```python
from build123d import *

# Parameters (mm, degrees)
BOSS_EXTRUDE1_DEPTH = 12
SKETCH2_R           = 3.1
BOSS_EXTRUDE2_DEPTH = 15
CUT_EXTRUDE1_START  = -50
CUT_EXTRUDE1_DEPTH  = 50
CUT_EXTRUDE2_START  = -15
CUT_EXTRUDE2_DEPTH  = 15
SKETCH5_W           = 7
SKETCH5_H           = 112.5
CUT_EXTRUDE3_DEPTH  = 12
SKETCH6_R           = 5.15
CUT_EXTRUDE4_DEPTH  = 2
FILLET1_R           = 4
BOSS_EXTRUDE3_DEPTH = 10
SKETCH9_R           = 2.1
CUT_EXTRUDE5_DEPTH  = 7
BOSS_EXTRUDE4_DEPTH = 7
SKETCH11_W          = 3.391399245
SKETCH11_H          = 0.49647288
BOSS_EXTRUDE7_DEPTH = 7
BOSS_EXTRUDE8_DEPTH = 10


with BuildPart() as part:
    # Sketch1 → Boss-Extrude1 (new body)
    with BuildSketch(Plane.XY):
        with BuildLine():
            Line((-5.64516129, 102.580645161), (-5.64516129, -27.419354839))
            ThreePointArc((-5.64516129, -27.419354839), (1.85483871, -34.919354839), (9.35483871, -27.419354839))
            Line((9.35483871, -27.419354839), (9.35483871, 102.580645161))
            ThreePointArc((9.35483871, 102.580645161), (1.85483871, 110.080645161), (-5.64516129, 102.580645161))
        make_face()
    extrude(amount=BOSS_EXTRUDE1_DEPTH)

    # Sketch2 → Boss-Extrude2 (add)
    with BuildSketch(Plane.XY.offset(12)):
        with Locations(Location((1.85483871, -27.419354839, 0), (0, 0, 180))):
            Circle(SKETCH2_R)
    extrude(amount=BOSS_EXTRUDE2_DEPTH)

    # Sketch3 → Cut-Extrude1 (cut)
    with BuildSketch(Plane.XY.offset(27).offset(CUT_EXTRUDE1_START)):
        with BuildLine():
            Line((0.166644408, -24.819354839), (3.543033011, -24.819354839))
            ThreePointArc((3.543033011, -24.819354839), (1.85483871, -30.519354839), (0.166644408, -24.819354839))
        make_face()
    extrude(amount=CUT_EXTRUDE1_DEPTH, mode=Mode.SUBTRACT)

    # Sketch4 → Cut-Extrude2 (cut)
    with BuildSketch(Plane.XY.offset(27).offset(CUT_EXTRUDE2_START)):
        with BuildLine():
            Line((0.166644408, -24.819354839), (3.543033011, -24.819354839))
            ThreePointArc((3.543033011, -24.819354839), (1.85483871, -24.319354839), (0.166644408, -24.819354839))
        make_face()
    extrude(amount=CUT_EXTRUDE2_DEPTH, mode=Mode.SUBTRACT)

    # Sketch5 → Cut-Extrude3 (cut)
    with BuildSketch(Plane.XY.offset(12)):
        with Locations((1.85483871, 36.330645161)):
            Rectangle(SKETCH5_W, SKETCH5_H)
    extrude(amount=-CUT_EXTRUDE3_DEPTH, mode=Mode.SUBTRACT)

    # Sketch6 → Cut-Extrude4 (cut)
    with BuildSketch(Plane.ZY.offset(5.64516129)):
        with Locations(Location((6, 78.768969581, 0), (0, 0, 270))):
            Circle(SKETCH6_R)
        with Locations(Location((6, 53.768969581, 0), (0, 0, 270))):
            Circle(SKETCH6_R)
        with Locations(Location((6, 28.768969581, 0), (0, 0, 270))):
            Circle(SKETCH6_R)
    extrude(amount=-CUT_EXTRUDE4_DEPTH, mode=Mode.SUBTRACT)

    # Fillet1
    # the kernel refuses this fillet: 4 mm, written as the material it adds along each edge
    with BuildSketch(Plane(origin=(-1.64516129, -19.919354839, 12), x_dir=(0, 1, 0), z_dir=(0, 0, -1)), Plane(origin=(5.35483871, -19.919354839, 12), x_dir=(-1, 0, 0), z_dir=(0, 0, -1)), Plane(origin=(5.35483871, 92.580645161, 12), x_dir=(0, -1, 0), z_dir=(0, 0, -1))) as fillet1_piece_1:
        with BuildLine():
            CenterArc((FILLET1_R, FILLET1_R), FILLET1_R, 180, 90)
            Line((0, FILLET1_R), (0, 0))
            Line((0, 0), (FILLET1_R, 0))
        make_face()
    extrude(amount=12)
    with BuildSketch(Plane(origin=(-1.64516129, 92.580645161, 12), x_dir=(0, -1, 0), z_dir=(0, 0, -1))) as fillet1_piece_2:
        with BuildLine():
            CenterArc((FILLET1_R, -FILLET1_R), FILLET1_R, 90, 90)
            Line((0, -FILLET1_R), (0, 0))
            Line((0, 0), (FILLET1_R, 0))
        make_face()
    extrude(amount=12)

    # Sketch7 → Boss-Extrude3 (add)
    with BuildSketch(Plane.XY.offset(12)):
        with BuildLine():
            ThreePointArc((-5.64516129, -27.419354839), (1.85483871, -34.919354839), (9.35483871, -27.419354839))
            ThreePointArc((9.35483871, -27.419354839), (1.85483871, -19.919354839), (-5.64516129, -27.419354839))
        make_face()
    extrude(amount=BOSS_EXTRUDE3_DEPTH)

    # Sketch9 → Cut-Extrude5 (cut)
    with BuildSketch(Plane.XY.offset(22)):
        with Locations((1.85483871, -27.419354839)):
            Circle(SKETCH9_R)
    extrude(amount=-CUT_EXTRUDE5_DEPTH, mode=Mode.SUBTRACT)

    # Sketch10 → Boss-Extrude4 (add)
    with BuildSketch(Plane.XY.offset(22)):
        with BuildLine():
            Line((0.694020033, -25.669354839), (3.015657386, -25.669354839))
            ThreePointArc((3.015657386, -25.669354839), (1.85483871, -25.319354839), (0.694020033, -25.669354839))
        make_face()
    extrude(amount=-BOSS_EXTRUDE4_DEPTH)

    # Sketch11 → Boss-Extrude7 (add)
    with BuildSketch(Plane.XY.offset(22)):
        with Locations((1.841860982, -25.665070635)):
            Rectangle(SKETCH11_W, SKETCH11_H)
    extrude(amount=-BOSS_EXTRUDE7_DEPTH)

    # Sketch12 → Boss-Extrude8 (add)
    with BuildSketch(Plane.XY.offset(22)):
        with BuildLine():
            Line((0.39134285, -25.913307075), (3.31833457, -25.913307075))
            ThreePointArc((3.31833457, -25.913307075), (1.85483871, -29.519354839), (0.39134285, -25.913307075))
        make_face()
        with BuildLine():
            Line((3.281340981, -26.003307075), (0.428336439, -26.003307075))
            ThreePointArc((0.428336439, -26.003307075), (1.85483871, -29.429354839), (3.281340981, -26.003307075))
        make_face(mode=Mode.SUBTRACT)
    extrude(amount=-BOSS_EXTRUDE8_DEPTH)


solid = part.part
```
Here's how the part is built. I have some questions about the finished solid (model axes, mm). A direction names the side the tool comes from. Round coordinates to 2 decimals unless told otherwise and drop trailing zeros. Write each loop counter-clockwise with the first axis right and the second up, starting at its lowest first coordinate (ties: lowest second). Pieces come first, ordered by that corner, then holes.
Q1. If we section it at B-B on z = 6: Write out the boundary of the cut face in (x, y), plus the area to 3 significant figures.
Q2. Which directions (+Z, -Z, +X, -X, +Y, -Y) give clear straight access to the entire face, cutting with the end or side of a thin tool? Please do faces 5 (the flat face through (5.355, 36, 6)), 6 (the flat face through (2, -28, 12)), 7 (the cylindrical face through (-4.659, 58.914, 6.226)), 8 (the cylindrical face through (0.23, -34.74, 13.29)), 9 (the flat face through (-5.645, 38, 6)).
Q3. If we mould it in two halves opening along Z, with no side actions, what happens to faces 1 (the cylindrical face through (1.966, -30.517, 5.916)), 2 (the flat face through (2, -28, 15)), 3 (the cylindrical face through (-4.66, 32.86, 2.87)), 4 (the cylindrical face through (-4.659, 83.914, 6.226))? For each: +Z half, -Z half, draft (parallel to the pull), parting line (faces both ways), or undercut.
Q4. If we section it at D-D on x = 6.75: Write out the boundary of the cut face in (y, z).
Q5. If we section it at C-C on z = 18.25: Write out the boundary of the cut face in (x, y).
Q6. Will these pins go through, and if not, where does the flat tip stop? P1, Ø1, axis at x = -2.5, z = 3, coming from the +Y side; P2, Ø2, axis at x = 0.5, z = 17.5, coming from the +Y side; P3, Ø3, axis at x = 3, y = -27.5, coming from the -Z side.
Q7. Please list where these lines run through material, in increasing order: probe 1 along Y at (x, z) = (2, 6.25); probe 2 along X at (y, z) = (60, 2.5); probe 3 along Y at (x, z) = (1.5, 10.5).
Q8. If we section it at A-A on y = 61.5: Write out the boundary of the cut face in (x, z), plus the area to 3 significant figures.
Answer below:
1. outline: (-5.65, -27.42) arc R7.5 ccw to (9.35, -27.42) - (9.35, 102.58) arc R7.5 ccw to (-5.65, 102.58) - (-5.65, 83.92) - (-3.65, 83.92) - (-3.65, 73.62) - (-5.65, 73.62) - (-5.65, 58.92) - (-3.65, 58.92) - (-3.65, 48.62) - (-5.65, 48.62) - (-5.65, 33.92) - (-3.65, 33.92) - (-3.65, 23.62) - (-5.65, 23.62) - close; hole (-1.65, -15.92) arc R4 ccw to (1.85, -19.89) arc R4 ccw to (5.35, -15.92) - (5.35, 88.58) arc R4 ccw to (1.85, 92.55) arc R4 ccw to (-1.65, 88.58) - close; hole (0.17, -24.82) arc R3.1 ccw (long way) to (3.54, -24.82) - close
1. area: 1,260 mm2
2. face 5: +Z, -Z
2. face 6: -Z
2. face 7: -X
2. face 8: +Z
2. face 9: +Z, -Z, -X, +Y, -Y
3. face 1: draft
3. face 2: +Z half
3. face 3: undercut
3. face 4: undercut
4. outline: (-33.1, 0) - (108.26, 0) - (108.26, 12) - (-21.74, 12) - (-21.74, 22) - (-33.1, 22) - close
5. outline: circle Ø15 at (1.85, -27.42); hole (0.43, -26) arc R2.01 ccw (long way) to (3.28, -26) - close
6. P1: stops at y = 109.01
6. P2: stops at y = -19.93
6. P3: stops at z = 12
7. probe 1: y = -34.92 to -30.52, -24.82 to -19.87, 92.53 to 110.08
7. probe 2: x = -5.65 to -1.65, 5.35 to 9.35
7. probe 3: y = -34.91 to -30.5, -24.82 to -19.83, 92.49 to 110.07
8. outline: (-5.65, 0) - (-1.65, 0) - (-1.65, 12) - (-5.65, 12) - close; (5.35, 0) - (9.35, 0) - (9.35, 12) - (5.35, 12) - close
8. area: 96.0 mm2
